Geometry: final body of the model. Coordinates: model frame, mm. Give positions to 0.01 mm unless a question says otherwise; leave off trailing zeros. Loops run counter-clockwise (first coordinate to the right, second up) from the corner with the lowest first, then second, coordinate; pieces in that order, holes last. Notation, with made-up numbers: (9.25, 68) - (60.25, 68) arc R7 ccw to (60.25, 76) - close; hole circle Ø7 at (-38.75, -13). An arc over 180 degrees is marked (long way). Use one line per item in the form item = value.
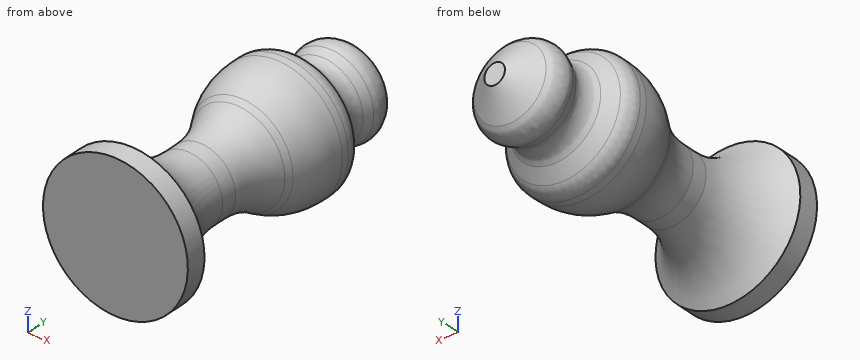
```python
from build123d import *

# Parameters (mm, degrees)
F3_R = 1.27


# Not quite as in the source:
# - a fillet or chamfer that OpenCascade refuses, or shapes differently, is made with other operations: its cross-section is extruded or revolved along the edge and cut away or added


with BuildPart() as f1:
    # F0 (on Right) → F1 (revolve)
    with BuildSketch(Plane.YZ):
        Polygon((-19.05, 0), (0, 0), (0, 0.635), (-1.7329187831, 3.0259732157), (-4.0311289486, 2.1315128542), (-5.611469965, 3.9772258134), (-8.1580255717, 3.9772258134), (-11.0198768943, 2.1315128542), (-17.4555711955, 2.1315128542), (-17.78, 4.4826099296), (-19.05, 4.4826099296), align=None)
    revolve(axis=Axis((0, -9.525, 0), (0, -1, 0)))

    # F2: fillet of radius 5.08 on 3 edges, made by hand

    # F2_s1 → F2_t2 (revolve)
    with BuildSketch(Plane.YZ):
        with BuildLine():
            ThreePointArc((-9.7626119553, 2.94236916), (-11.0808174663, 2.3384414426), (-12.5159394181, 2.1315128542))
            Line((-12.5159394181, 2.1315128542), (-11.0198768943, 2.1315128542))
            Line((-11.0198768943, 2.1315128542), (-9.7626119553, 2.94236916))
        make_face()
    revolve(axis=Axis((0, -11.0198768943, 0), (0, -1, 0)))

    # F2_s3 → F2_t4 (revolve, cut)
    with BuildSketch(Plane.YZ):
        with BuildLine():
            ThreePointArc((-9.4152905107, 3.1663695077), (-8.0970849997, 3.7702972251), (-6.6619630479, 3.9772258134))
            Line((-6.6619630479, 3.9772258134), (-8.1580255717, 3.9772258134))
            Line((-8.1580255717, 3.9772258134), (-9.4152905107, 3.1663695077))
        make_face()
    revolve(axis=Axis((0, -8.1580255717, 0), (0, -1, 0)), mode=Mode.SUBTRACT)

    # F2_s5 → F2_t6 (revolve)
    with BuildSketch(Plane.YZ):
        with BuildLine():
            ThreePointArc((-17.78, 4.4826099296), (-15.9389265067, 2.7579060655), (-13.495202592, 2.1315128542))
            Line((-13.495202592, 2.1315128542), (-17.4555711955, 2.1315128542))
            Line((-17.4555711955, 2.1315128542), (-17.78, 4.4826099296))
        make_face()
    revolve(axis=Axis((0, -17.4555711955, 0), (0, -1, 0)))

    # F3
    f3_edges = [f1.edges().sort_by_distance(p)[0] for p in [
        (0, -5.61147, -3.977226),
        (0, -4.031129, -2.131513),
        (0, -1.732919, -3.025973),
    ]]
    fillet(f3_edges, radius=F3_R)


solid = f1.part
```
(1) Cut plane B-B (y = -14.5). Return the cut outline in (x, z).
Solution:
outline = circle Ø4.46 at (0, 0)
(2) Pin query (flat end, axial travel): P1, Ø5, axis at x = 3, y = -7.5, coming from the -Z side; P2, Ø2, axis at x = 2.5, z = -2, coming from the +Y side; P3, Ø2, axis at x = 0.5, y = -13, coming from the -Z side. Return the tip coordinate at first contact, or that it passes through.
Solution:
P1 = -3.93
P2 = -1.14
P3 = -2.15
(3) Cut plane A-A (y = -12). Return the cut outline in (x, z), plus the area to 3 significant figures.
Solution:
outline = circle Ø4.32 at (0, 0)
area = 14.6 mm2
(4) Material intervals for L1, parallel to Y at x = -2.75, z = 1.25; L2, parallel to Y at x = -0.25, z = 3.5; L3, parallel to Y at x = 2, z = 3.75, sorted ascending. Write a range as from..to.
Solution:
L1 = -19.05..-16.37, -9.64..-4.79
L2 = -19.05..-16.97, -8.79..-5.21
L3 = -19.05..-17.62
